Model file for the job. Use its own axes, mm. A direction names the side the tool comes from. Round coordinates to 2 decimals unless told otherwise and drop trailing zeros. Order: outer loops, then holes, each group sorted by start corner. A loop starts at its lowest first (then second) coordinate and runs counter-clockwise, first axis right, second up. Notation, with made-up numbers: (9, -34.75) - (52, -34.75) arc R8 cw to (52, -29.75) - close; hole circle Ø8 at (69.5, 67). An arc over 180 degrees is marked (long way). Use one line per item in the form item = value.
from build123d import *

# Parameters (mm, degrees)
F0_W      = 22.25
F0_H      = 17.875
F1_DEPTH  = 3.175
F2_DEPTH  = 5.08
F3_DEPTH  = 2.54
F4_DEPTH  = 5.08
F5_DEPTH  = 5.08
F6_DEPTH  = 5.08
F7_DEPTH  = 4.7498
F8_DEPTH  = 4.7498
F9_DEPTH  = 4.7498
F10_DEPTH = 4.7498
F11_DEPTH = 2.54
F12_R     = 1.325
F13_DEPTH = 25.4
F14_DEPTH = 25.4
F15_DEPTH = 25.4
F16_DEPTH = 25.4


# Not quite as in the source:
# - a feature names something its author has since deleted; it is built from what else it names


with BuildPart() as f1:
    # F0 (on Top) → F1 (new body)
    with BuildSketch(Plane.XY):
        Polygon((0, 35.75), (0, 0), (44.5, 0), (44.5, 35.75), (64.5, 35.75), (64.5, 39.25), (64.5, 42.75), (44.5, 42.75), (44.5, 78.5), (0, 78.5), (0, 42.75), (-20, 42.75), (-20, 39.25), (-20, 35.75), align=None)
        with Locations((22.25, 17.875)):
            Rectangle(F0_W, F0_H, mode=Mode.SUBTRACT)
        with Locations((22.25, 60.625)):
            Rectangle(F0_W, F0_H, mode=Mode.SUBTRACT)
    extrude(amount=F1_DEPTH)

    # F2 (add): a face of the model
    f2_faces = [f1.faces().sort_by_distance(p)[0] for p in [
        (22.25, 69.5625, 1.5875),
    ]]
    extrude(f2_faces, amount=F2_DEPTH)

    # F3 (add): faces of the model
    f3_faces = [f1.faces().sort_by_distance(p)[0] for p in [
        (22.25, 51.6875, 1.5875),
        (22.25, 26.8125, 1.5875),
    ]]
    extrude(f3_faces, amount=F3_DEPTH, dir=(0, 1, 0))

    # F4 (add): a face of the model
    f4_faces = [f1.faces().sort_by_distance(p)[0] for p in [
        (22.25, 8.9375, 1.5875),
    ]]
    extrude(f4_faces, amount=F4_DEPTH)

    # F5 (add): faces of the model
    f5_faces = [f1.faces().sort_by_distance(p)[0] for p in [
        (33.375, 59.355, 1.5875),
        (33.375, 20.415, 1.5875),
    ]]
    extrude(f5_faces, amount=F5_DEPTH)

    # F6 (add): faces of the model
    f6_faces = [f1.faces().sort_by_distance(p)[0] for p in [
        (11.125, 59.355, 1.5875),
        (11.125, 20.415, 1.5875),
    ]]
    extrude(f6_faces, amount=F6_DEPTH)

    # F7 (cut): faces of the model
    f7_faces = [f1.faces().sort_by_distance(p)[0] for p in [
        (44.5, 60.625, 1.5875),
        (44.5, 17.875, 1.5875),
    ]]
    extrude(f7_faces, amount=-F7_DEPTH, mode=Mode.SUBTRACT)

    # F8 (cut): faces of the model
    f8_faces = [f1.faces().sort_by_distance(p)[0] for p in [
        (0, 60.625, 1.5875),
        (0, 17.875, 1.5875),
    ]]
    extrude(f8_faces, amount=-F8_DEPTH, mode=Mode.SUBTRACT)

    # F9 (cut): a face of the model
    f9_faces = [f1.faces().sort_by_distance(p)[0] for p in [
        (-20, 39.25, 1.5875),
    ]]
    extrude(f9_faces, amount=-F9_DEPTH, mode=Mode.SUBTRACT)

    # F10 (cut): a face of the model
    f10_faces = [f1.faces().sort_by_distance(p)[0] for p in [
        (64.5, 39.25, 1.5875),
    ]]
    extrude(f10_faces, amount=-F10_DEPTH, mode=Mode.SUBTRACT)

    # F11 (cut): a face of the model
    f11_faces = [f1.faces().sort_by_distance(p)[0] for p in [
        (22.25, 64.4825, 1.5875),
    ]]
    extrude(f11_faces, amount=-F11_DEPTH, mode=Mode.SUBTRACT)

    # F12 (on face) → F13 (cut)
    with BuildSketch(Plane(origin=(0, 0, 0), x_dir=(1, 0, 0), z_dir=(0, 0, -1))):
        with BuildLine():
            ThreePointArc((34.6002, -74.675), (35.9252, -76), (37.2502, -74.675))
            ThreePointArc((37.2502, -74.675), (35.9252, -73.35), (34.6002, -74.675))
        make_face()
        with Locations((8.5748, -74.675)):
            Circle(F12_R)
        with Locations((8.5748, -39.25)):
            Circle(F12_R)
        with BuildLine():
            ThreePointArc((34.6002, -39.25), (35.9252, -40.575), (37.2502, -39.25))
            ThreePointArc((37.2502, -39.25), (35.9252, -37.925), (34.6002, -39.25))
        make_face()
        with Locations((35.9252, -3.825)):
            Circle(F12_R)
        with Locations((8.5748, -3.825)):
            Circle(F12_R)
    extrude(amount=-F13_DEPTH, mode=Mode.SUBTRACT)

    # F12 (on face) → F14 (cut)
    with BuildSketch(Plane(origin=(0, 0, 0), x_dir=(1, 0, 0), z_dir=(0, 0, -1))):
        with Locations((22.25, -74.675)):
            Circle(F12_R)
    extrude(amount=-F14_DEPTH, mode=Mode.SUBTRACT)

    # F12 (on face) → F15 (cut)
    with BuildSketch(Plane(origin=(0, 0, 0), x_dir=(1, 0, 0), z_dir=(0, 0, -1))):
        with Locations((22.25, -7.00875)):
            Circle(F12_R)
        with Locations((22.25, -46.73875)):
            Circle(F12_R)
    extrude(amount=-F15_DEPTH, mode=Mode.SUBTRACT)

    # F12 (on face) → F16 (cut)
    with BuildSketch(Plane(origin=(0, 0, 0), x_dir=(1, 0, 0), z_dir=(0, 0, -1))):
        with Locations((22.25, -33.03125)):
            Circle(F12_R)
    extrude(amount=-F16_DEPTH, mode=Mode.SUBTRACT)


solid = f1.part
(1) Slice it at D-D on x = 8.5. Give the cut face in (y, z) (3 decimals).
Report:
outline = (0, 0) - (2.502, 0) - (2.502, 3.175) - (0, 3.175) - close; (5.148, 0) - (37.927, 0) - (37.927, 3.175) - (5.148, 3.175) - close; (40.573, 0) - (73.352, 0) - (73.352, 3.175) - (40.573, 3.175) - close; (75.998, 0) - (78.5, 0) - (78.5, 3.175) - (75.998, 3.175) - close
(2) Slice it at A-A on y = 25. Give the cut face in (x, z) (3 decimals).
Report:
outline = (4.75, 0) - (16.205, 0) - (16.205, 3.175) - (4.75, 3.175) - close; (28.295, 0) - (39.75, 0) - (39.75, 3.175) - (28.295, 3.175) - close
(3) Pin check, flat tips, straight feed: pin 1 (12 mm diameter, centred on x = -2.5, y = 47, fed in from +Z) (3 decimals); pin 2 (1 mm diameter, centred on x = -4, z = 1.5, fed in from -Y); pin 3 (1 mm diameter, centred on y = 65, z = 2, fed in from +X); pin 4 (1.6 mm diameter, centred on y = 17, z = 1.5, fed in from -X). Stop position of each tip, or through.
Report:
pin_1 = 3.175
pin_2 = 35.75
pin_3 = 39.75
pin_4 = 4.75
(4) Slice it at B-B on x = 22.25. Count the separate pieces of the cut face and the enclosed holes in it, then the cut area to 3 significant figures.
Report:
separate_pieces = 7
enclosed_holes = 0
area = 134 mm2
(5) Pull direction Y, two halves, no side cores. Call faces 5 (the face through (39.75, 18, 2)), 6 (the face through (-5, 42.75, 2)), 7 (the face through (21.273, 6.113, 1.565)), 8 (the face through (21.96, 48.03, 1.57)): released by +Y, released by -Y, zero draft, split by the parting line, or undercut.
Report:
face_5 = zero draft
face_6 = released by +Y
face_7 = undercut
face_8 = undercut
(6) Tool access for faces 1 (the face through (39.75, 60, 2)), 2 (the face through (-5, 35.75, 2)), 3 (the face through (4.75, 61, 2)), 4 (the face through (22, 54.228, 2)): list every direction of +Z, -Z, +X, -X, +Y, -Y with a clear straight run to the whole face (end or side of a thin tool).
Report:
face_1 = +Z, -Z, +X, +Y
face_2 = +Z, -Z, -X, -Y
face_3 = +Z, -Z, -X, +Y
face_4 = +Z, -Z
(7) Probe probe 1 along X at (y, z) = (39.25, 1.45); probe 2 along Y at (x, z) = (9.5, 2.7); probe 3 along X at (y, z) = (57, 2.45) (3 decimals). List the from-to ranges inside material, lowest first. Write a range as [from, to].
Report:
probe_1 = [-15.25, 7.25], [9.9, 34.6], [37.25, 59.75]
probe_2 = [0, 2.88], [4.77, 38.3], [40.2, 73.73], [75.62, 78.5]
probe_3 = [4.75, 16.205], [28.295, 39.75]
(8) Slice it at C-C on y = 39.25. Give the cut face in (x, z) (3 decimals).
Report:
outline = (-15.25, 0) - (7.25, 0) - (7.25, 3.175) - (-15.25, 3.175) - close; (9.9, 0) - (34.6, 0) - (34.6, 3.175) - (9.9, 3.175) - close; (37.25, 0) - (59.75, 0) - (59.75, 3.175) - (37.25, 3.175) - close
